The model under review builds one solid part; all positions refer to its coordinate system, in mm. A direction names the side the tool comes from. Give positions to 0.01 mm unless a question says otherwise; leave off trailing zeros. Loops run counter-clockwise (first coordinate to the right, second up) from the corner with the lowest first, then second, coordinate; pieces in that order, holes last. Notation, with made-up numbers: M -20.75,44.25 L 22.25,44.25 A29 cw 22.25,71.25 Z; hole C 6.5,41 d9. An arc over 180 degrees is marked long. Write item = value, one per line. Start each with the question number.
1. Wall thickness on line 1 along Y through (x, z) = (1, 37.5); line 2 along Y through (x, z) = (14, 30.5); line 3 along Y through (x, z) = (15.5, 43): over which ranges is each line inside the solid? List them lowest first. Write a range as from..to.
2. For pin 1 (15.5 mm diameter, centred on x = 17, y = 2, fed in from +Z); pin 2 (2 mm diameter, centred on x = 9, z = -1.5, fed in from +Y); pin 3 (2 mm diameter, centred on y = -3.5, z = 8.5, fed in from -X); pin 4 (1 mm diameter, centred on x = 21, y = 2.5, fed in from +Z), all flat-tipped, find the tip position at first contact; note any pin that passes through.
3. We need section D-D on z = 65.5. Give the boundary of the cut face in (x, y), then the cut area to 3 significant figures.
4. We need section A-A on z = 11. Give the boundary of the cut face in (x, y).
5. We need section C-C on x = -1. Give the boundary of the cut face in (y, z).
6. Draft analysis for pull direction X (two halves, no side actions). For faces 1 (the face through (9, 13, 29)), 2 (the face through (-11.697, -0.257, 33.341)), 3 (the face through (9, -4, 0)), state which applies: pulls with the +X half, pulls with the -X half, needs draft (parallel to the pull), parting line crosses it, or undercut.
7. We need section B-B on y = 0. Give the boundary of the cut face in (x, z), then the cut area to 3 significant figures.
8. For faces 4 (the face through (9, -9.7, 35)), 5 (the face through (-3, 0, -1)), 6 (the face through (9, -11.7, 33)), list the 3-axis set-ups (+Z, -Z, +X, -X, +Y, -Y) from which the entire face can be reached by the end or side of a thin tool; tool diameter is ignored.
from build123d import *

# Parameters (mm, degrees)
Y_KSEKLIK_EKSTR_ZYON1_DEPTH = 70.2
Y_KSEKLIK_EKSTR_ZYON2_START = 2.5
Y_KSEKLIK_EKSTR_ZYON2_DEPTH = 2.5
Y_KSEKLIK_EKSTR_ZYON5_DEPTH = 40
PAH1_SIZE                   = 2.5
KES_EKSTR_ZYON1_DEPTH       = 10


with BuildPart() as part:
    # Çizim1 → Yükseklik-Ekstrüzyon1 (new body)
    with BuildSketch(Plane.XY):
        with BuildLine():
            Line((0, 11.7), (18.4, 11.7))
            ThreePointArc((18.4, 11.7), (30.1, 0), (18.4, -11.7))
            Line((18.4, -11.7), (0, -11.7))
            ThreePointArc((0, -11.7), (-11.7, 0), (0, 11.7))
        make_face()
        with BuildLine():
            ThreePointArc((0, 9.7), (-9.7, 0), (0, -9.7))
            Line((0, -9.7), (18.4, -9.7))
            ThreePointArc((18.4, -9.7), (28.1, 0), (18.4, 9.7))
            Line((18.4, 9.7), (0, 9.7))
        make_face(mode=Mode.SUBTRACT)
    extrude(amount=Y_KSEKLIK_EKSTR_ZYON1_DEPTH)

    # Çizim2 → Yükseklik-Ekstrüzyon2 (add)
    with BuildSketch(Plane(origin=(0, 0, 0), x_dir=(-1, 0, 0), z_dir=(0, 0, -1)).offset(Y_KSEKLIK_EKSTR_ZYON2_START)):
        with BuildLine():
            Line((0, 11.7), (-18.4, 11.7))
            ThreePointArc((-18.4, 11.7), (-30.1, 0), (-18.4, -11.7))
            Line((-18.4, -11.7), (0, -11.7))
            ThreePointArc((0, -11.7), (11.7, 0), (0, 11.7))
        make_face()
    extrude(amount=-Y_KSEKLIK_EKSTR_ZYON2_DEPTH)

    # Çizim8 → Yükseklik-Ekstrüzyon5 (add)
    with BuildSketch(Plane.XY.offset(70.2)):
        Polygon((14.7, 11.7), (3.7, 11.7), (1.2, 14.2), (17.2, 14.2), align=None)
    extrude(amount=-Y_KSEKLIK_EKSTR_ZYON5_DEPTH)

    # Pah1
    pah1_edges = [part.edges().sort_by_distance(p)[0] for p in [
        (9.2, 11.7, 30.2),
    ]]
    chamfer(pah1_edges, length=PAH1_SIZE - 0.0001)  # a hair under: the kernel refuses the full size

    # Çizim9 → Kes-Ekstrüzyon1 (cut)
    with BuildSketch(Plane(origin=(0, 0, -2.5), x_dir=(-1, 0, 0), z_dir=(0, 0, -1))):
        with BuildLine():
            Line((0, -3), (-18.4, -3))
            ThreePointArc((-18.4, -3), (-21.4, 0), (-18.4, 3))
            Line((-18.4, 3), (0, 3))
            ThreePointArc((0, 3), (3, 0), (0, -3))
        make_face()
    extrude(amount=-KES_EKSTR_ZYON1_DEPTH, mode=Mode.SUBTRACT)


solid = part.part
Final values:
q1.line_1 = -11.7..-9.7, 9.7..11.7
q1.line_2 = -11.7..-9.7, 9.7..14.2
q1.line_3 = -11.7..-9.7, 9.7..11.7, 12.5..14.2
q2.pin_1 = 70.2
q2.pin_2 = 11.7
q2.pin_3 = -11.43
q2.pin_4 = 0
q3.outline = M 0,-11.7 L 18.4,-11.7 A11.7 ccw 18.4,11.7 L 14.7,11.7 L 17.2,14.2 L 1.2,14.2 L 3.7,11.7 L 0,11.7 A11.7 ccw Z; hole M 0,-9.7 L 18.4,-9.7 A9.7 ccw 18.4,9.7 L 0,9.7 A9.7 ccw Z
q3.area = 242 mm²
q4.outline = M 0,-11.7 L 18.4,-11.7 A11.7 ccw 18.4,11.7 L 0,11.7 A11.7 ccw Z; hole M 0,-9.7 L 18.4,-9.7 A9.7 ccw 18.4,9.7 L 0,9.7 A9.7 ccw Z
q5.outline = M -11.66,-2.5 L -2.83,-2.5 L -2.83,0 L -9.65,0 L -9.65,70.2 L -11.66,70.2 Z; M 2.83,-2.5 L 11.66,-2.5 L 11.66,70.2 L 9.65,70.2 L 9.65,0 L 2.83,0 Z
q6.face_1 = needs draft
q6.face_2 = pulls with the -X half
q6.face_3 = undercut
q7.outline = M -11.7,-2.5 L -3,-2.5 L -3,0 L -9.7,0 L -9.7,70.2 L -11.7,70.2 Z; M 21.4,-2.5 L 30.1,-2.5 L 30.1,70.2 L 28.1,70.2 L 28.1,0 L 21.4,0 Z
q7.area = 324 mm²
q8.face_4 = +Z
q8.face_5 = +Z, -Z
q8.face_6 = +Z, -Z, +X, -X, -Y
